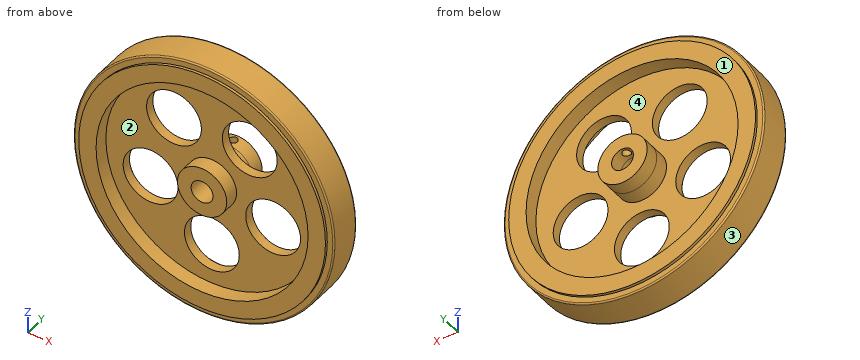
```python
from build123d import *

# Parameters (mm, degrees)
SKETCH_1_R          = 47.5
SKETCH_1_R_2        = 9
SKETCH_1_R_3        = 4
EXTRUDE_1_DEPTH     = 7
SKETCH_2_R          = 47.5
SKETCH_2_R_2        = 45
CUT_EXTRUDE_1_DEPTH = 1
SKETCH_3_R          = 38.66
SKETCH_3_R_2        = 9
CUT_EXTRUDE_2_DEPTH = 5.3
SKETCH_4_R          = 10
CUT_EXTRUDE_3_DEPTH = 9.7
FILLET_1_R          = 0.5
SKETCH_5_R          = 9
SKETCH_5_R_2        = 4
EXTRUDE_2_DEPTH     = 5.2
SKETCH_6_R          = 1.5
CUT_EXTRUDE_4_DEPTH = 48.5000001


with BuildPart() as part:
    # 草圖1 → 填料-伸長1 (new body, symmetric)
    with BuildSketch(Plane(origin=(0, 0, 0), x_dir=(1, 0, 0), z_dir=(0, 1, 0))):
        Circle(SKETCH_1_R)
        Circle(SKETCH_1_R_2, mode=Mode.SUBTRACT)
        Circle(SKETCH_1_R_2)
        Circle(SKETCH_1_R_3, mode=Mode.SUBTRACT)
    extrude(amount=EXTRUDE_1_DEPTH, both=True)

    # 草圖2 → 除料-伸長1 (cut)
    with BuildSketch(Plane(origin=(0, 7, 0), x_dir=(1, 0, 0), z_dir=(0, 1, 0))):
        Circle(SKETCH_2_R)
        Circle(SKETCH_2_R_2, mode=Mode.SUBTRACT)
    cut_extrude_1 = extrude(amount=-CUT_EXTRUDE_1_DEPTH, mode=Mode.SUBTRACT)

    # 鏡射1: 除料-伸長1 across plane
    add(cut_extrude_1.mirror(Plane.ZX), mode=Mode.SUBTRACT)

    # 草圖3 → 除料-伸長2 (cut)
    with BuildSketch(Plane(origin=(0, 7, 0), x_dir=(1, 0, 0), z_dir=(0, 1, 0))):
        Circle(SKETCH_3_R)
        Circle(SKETCH_3_R_2, mode=Mode.SUBTRACT)
    cut_extrude_2 = extrude(amount=-CUT_EXTRUDE_2_DEPTH, mode=Mode.SUBTRACT)

    # 鏡射2: 除料-伸長2 across plane
    add(cut_extrude_2.mirror(Plane.ZX), mode=Mode.SUBTRACT)

    # 草圖4 → 除料-伸長3 (cut, through all)
    with BuildSketch(Plane(origin=(0, 1.7, 0), x_dir=(1, 0, 0), z_dir=(0, 1, 0))):
        with Locations((0, 23.5)):
            Circle(SKETCH_4_R)
        with Locations((22.349828133, 7.261899368)):
            Circle(SKETCH_4_R)
        with Locations((13.812953429, -19.011899368)):
            Circle(SKETCH_4_R)
        with Locations((-13.812953429, -19.011899368)):
            Circle(SKETCH_4_R)
        with Locations((-22.349828133, 7.261899368)):
            Circle(SKETCH_4_R)
    extrude(amount=-CUT_EXTRUDE_3_DEPTH, mode=Mode.SUBTRACT)

    # 圓角1
    fillet_1_edges = [part.edges().sort_by_distance(p)[0] for p in [
        (-47.5, 6, 0),
        (-47.5, -6, 0),
    ]]
    fillet(fillet_1_edges, radius=FILLET_1_R)

    # 草圖5 → 填料-伸長2 (add)
    with BuildSketch(Plane(origin=(0, 7, 0), x_dir=(1, 0, 0), z_dir=(0, 1, 0))):
        Circle(SKETCH_5_R)
        Circle(SKETCH_5_R_2, mode=Mode.SUBTRACT)
    extrude(amount=EXTRUDE_2_DEPTH)

    # 草圖6 → 除料-伸長4 (cut, through all)
    with BuildSketch(Plane.XY):
        with Locations((0, 9.9)):
            Circle(SKETCH_6_R)
    extrude(amount=CUT_EXTRUDE_4_DEPTH, mode=Mode.SUBTRACT)


solid = part.part
```
Verification items for the finished model (mm, model axes). Face numbers are marked on the shaded views. Give positions to 0.01 mm unless a question says otherwise; leave off trailing zeros. Order: outer loops, then holes, each group sorted by start corner. A loop starts at its lowest first (then second) coordinate and runs counter-clockwise, first axis right, second up. Notation, with made-up numbers: (72, 78) - (127, 78) arc R34 ccw to (127, 111) - close; hole circle Ø2 at (23, 21.5). An arc over 180 degrees is marked (long way). Answer as CSV lines item,"result". Start each with the question number.
Item 1: Section check A-A, the plane x = 0. State how many separate pieces and enclosed holes the cut face has, plus the area to 3 significant figures.
Item 2: Mould release check, pull along X, two halves, no side actions. Record for the marked faces 1, 2, 3 and 4: released by +X, released by -X, zero draft, split by the parting line, or undercut.
Item 3: Section check D-D, the plane y = 9.9. Record the boundary of the cut face in (x, z).
Item 4: Gauge pin test, flat ends, axial feed: pin 1 (4 mm diameter, centred on x = 23.5, y = 6.5, fed in from +Z); pin 2 (3 mm diameter, centred on x = -30.5, z = -14.5, fed in from -Y); pin 3 (1.8 mm diameter, centred on x = 0, y = 9.9, fed in from +Z). Record the tip position at first contact, or that the pin passes through.
Item 5: Material ranges on L1, parallel to X at y = -5.25, z = 0; L2, parallel to Y at x = 0, z = 7, recorded low to high.
Filled in:
1,separate pieces,"4"
1,enclosed holes,"0"
1,area,"548 mm^2"
2,face 1,"zero draft"
2,face 2,"undercut"
2,face 3,"split by the parting line"
2,face 4,"undercut"
3,outline,"(-1.5, 3.71) - (-1.5, 8.87) arc R9 ccw (long way) to (1.5, 8.87) - (1.5, 3.71) arc R4 cw (long way) to start"
4,pin 1,"z = 42.24"
4,pin 2,"y = -1.7"
4,pin 3,"z = -3.9"
5,L1,"-47.5 to -38.66, -9 to -4, 4 to 9, 38.66 to 47.5"
5,L2,"-7 to 8.4, 11.4 to 12.2"
